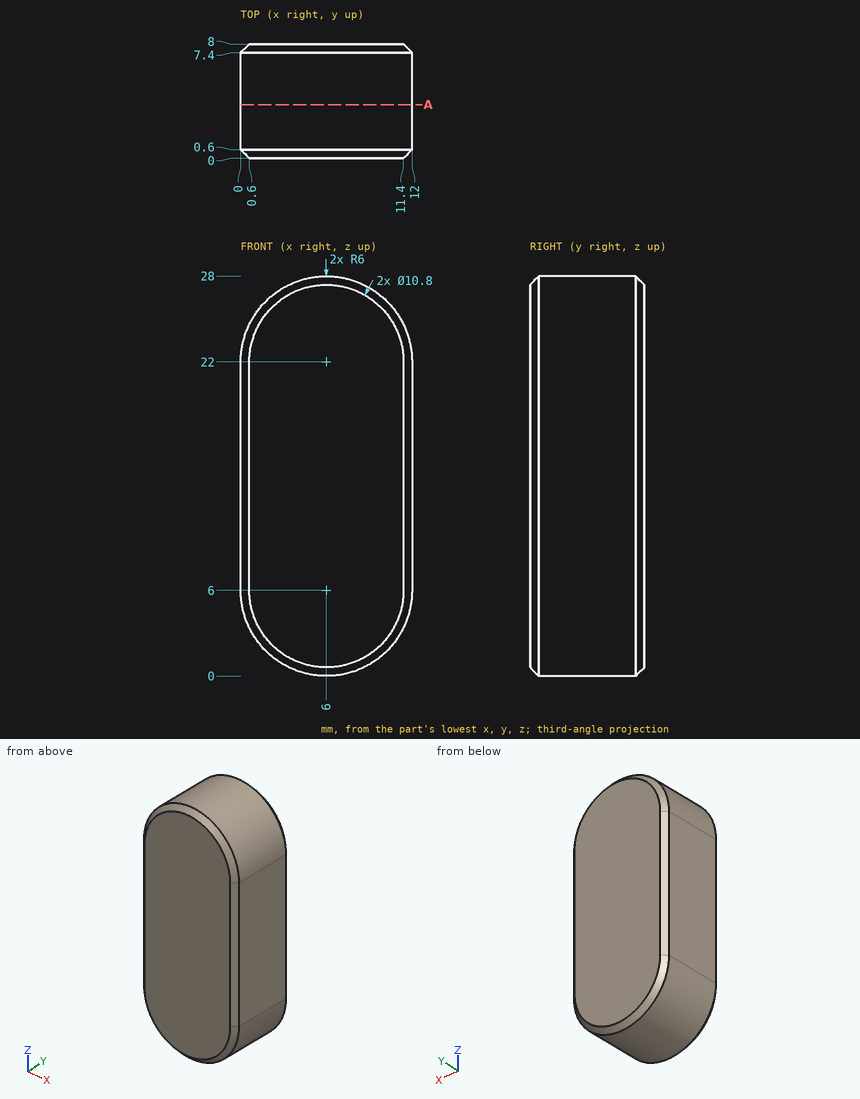
The drawing under review shows one solid part. Ordinate dimensions are in mm from its lowest x, y, z. Coordinates: 2 decimals unless noted, no trailing zeros. Write each loop counter-clockwise with the first axis right and the second up, starting at its lowest first coordinate (ties: lowest second). Pieces come first, ordered by that corner, then holes. Notation, with made-up numbers: M -10.5,81.5 L 3.5,81.5 A22 cw 3.5,88.5 Z; hole C -8,2.25 d11. An arc over 180 degrees is marked long. Answer as a JSON object with one key per item and string values.
Item 1: Add section A-A, the plane y = 3.75. Give the boundary of the cut face in (x, z), and give its area (3 significant figures).
Outcome:
{"outline": "M 0,6 A6 ccw 12,6 L 12,22 A6 ccw 0,22 Z", "area": "305 mm²"}
Item 2: Wall thickness on probe 1 along Z at (x, y) = (4.5, 1.25); probe 2 along X at (y, z) = (2.5, 3); probe 3 along Z at (x, y) = (9.75, 3.25): over which ranges is each line inside the solid? List them lowest first.
Outcome:
{"probe 1": "0.19 to 27.81", "probe 2": "0.8 to 11.2", "probe 3": "1.32 to 26.68"}
Item 3: Insertion check: pin 1 Ø1.5 at (x, y) = (8, 4) entering from -Z; pin 2 Ø3 at (x, y) = (3, 5.5) entering from +Z; pin 3 Ø2 at (x, y) = (10, 3.5) entering from +Z. Each pin has a flat end and moves straight along its axis. Give the tip position at first contact, or say it passes through.
Outcome:
{"pin 1": "z = 0.13", "pin 2": "z = 27.81", "pin 3": "z = 27.2"}
